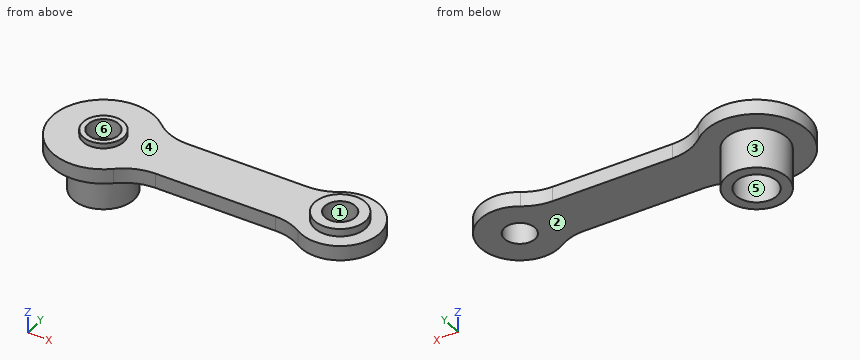
Autodesk Inventor part; units mm, degrees
ref_plane "YZ Plane" through (0, 0, 0) normal (1, 0, 0) x (0, 1, 0)
ref_plane "XZ Plane" through (0, 0, 0) normal (0, 1, 0) x (-1, 0, 0)
ref_plane "XY Plane" through (0, 0, 0) normal (0, 0, 1) x (1, 0, 0)
sketch "Base" plane through (0, 0, 0) normal (0, 0, 1) x (1, 0, 0)
  circle A0 centre (0, 0) radius 10
  line L0 (0, 0) -> (46, 0) construction
  circle A1 centre (46, 0) radius 7.75
  line L1 (8.6603, 5) -> (40.0786, 5)
  line L2 (40.0786, 5) -> (40.0786, -5)
  line L3 (40.0786, -5) -> (8.6603, -5)
  line L4 (8.6603, -5) -> (8.6603, 5)
  circle A2 centre (46, 0) radius 3
  circle A3 centre (0, 0) radius 3
  point P0 (8.6603, 0)
  point P1 (8.6603, -5)
  dimension "d0" = 20
  dimension "d2" = 15.5
  dimension "d1" = 46
  dimension "d3" = 10
  dimension "d4" = 6
  dimension "d5" = 6
extrude "Plate1" add sketch "Base" along normal blind 2.9
sketch "Shoulder" plane through (0, 0, 0) normal (0, 0, -1) x (-1, 0, 0)
  circle A0 centre (0, 0) radius 3
  circle A1 centre (0, 0) radius 3
  circle A2 centre (0, 0) radius 6
  circle A3 centre (0, 0) radius 4
  dimension "d7" = 12
  dimension "d8" = 2
extrude "ShoulderFeature" add sketch "Shoulder" along normal blind 8 contours A2
sketch "Mount" plane through (0, 0, 2.9) normal (0, 0, 1) x (1, 0, 0)
  circle A0 centre (46, 0) radius 3
  circle A1 centre (46, 0) radius 5
  point P0 (0, 0)
  dimension "d11" = 2
extrude "MountFeature" add sketch "Mount" along normal blind 1.5
fillet "BaseFilletsFeature" radius 10 2 edges at (8.6603, 5, 1.45) (8.6603, -5, 1.45)
fillet "EndFilletsFeature" radius 10 2 edges at (40.0786, 5, 1.45) (40.0786, -5, 1.45)
sketch "Sketch6" plane through (0, 0, 2.9) normal (0, 0, 1) x (1, 0, 0)
  circle A0 centre (0, 0) radius 3
  circle A1 centre (0, 0) radius 4
  dimension "d17" = 1
extrude "Extrusion3" add sketch "Sketch6" along normal blind 1
equation "\"d6\" = Thickness"
equation "\"BendRadius\" = Thickness"
equation "\"BendReliefWidth\" = Thickness"
equation "\"BendReliefDepth\" = 0.5 * Thickness"
equation "\"CornerReliefSize\" = 4 * Thickness"
equation "\"MinimumRemnant\" = 2 * Thickness"
equation "\"TransitionRadius\" = BendRadius"
equation "\"JacobiRadiusSize\" = BendRadius"
equation "\"GapSize\" = Thickness"
properties part number "LegChainTensionerArm"
CAD build for the part. Positions are in the model's coordinates, mm. Face numbers are marked on the shaded views. A direction names the side the tool comes from. Coordinates: 2 decimals unless noted, no trailing zeros. Order: outer loops, then holes, each group sorted by start corner. A loop starts at its lowest first (then second) coordinate and runs counter-clockwise, first axis right, second up.
Item 1: Band-saw the part on A-A on x = 46. List the corners of the cut face in (y, z), plus the area to 4 significant figures.
Check sheet entries:
outline: (-7.75, 0) - (-3, 0) - (-3, 4.4) - (-5, 4.4) - (-5, 2.9) - (-7.75, 2.9) - close; (3, 0) - (7.75, 0) - (7.75, 2.9) - (5, 2.9) - (5, 4.4) - (3, 4.4) - close
area: 33.55 mm2
Item 2: Band-saw the part on D-D on x = 0. List the corners of the cut face in (y, z), plus the area to 3 significant figures.
Check sheet entries:
outline: (-10, 0) - (-6, 0) - (-6, -8) - (-4, -8) - (-4, 0) - (-3, 0) - (-3, 3.9) - (-4, 3.9) - (-4, 2.9) - (-10, 2.9) - close; (3, 0) - (4, 0) - (4, -8) - (6, -8) - (6, 0) - (10, 0) - (10, 2.9) - (4, 2.9) - (4, 3.9) - (3, 3.9) - close
area: 74.6 mm2
Item 3: Band-saw the part on B-B on y = 0. List the corners of the cut face in (x, z), plus the area to 3 significant figures.
Check sheet entries:
outline: (-10, 0) - (-6, 0) - (-6, -8) - (-4, -8) - (-4, 0) - (-3, 0) - (-3, 3.9) - (-4, 3.9) - (-4, 2.9) - (-10, 2.9) - close; (3, 0) - (4, 0) - (4, -8) - (6, -8) - (6, 0) - (43, 0) - (43, 4.4) - (41, 4.4) - (41, 2.9) - (4, 2.9) - (4, 3.9) - (3, 3.9) - close; (49, 0) - (53.75, 0) - (53.75, 2.9) - (51, 2.9) - (51, 4.4) - (49, 4.4) - close
area: 190 mm2
Item 4: Drill centre lines: L1, parallel to Y at x = 46, z = 1; L2, parallel to Y at x = 0, z = 0.85; L3, parallel to Z at x = 29, y = -4.5. Where is each one in solid material? Low to high.
Check sheet entries:
L1: y = -7.75 to -3, 3 to 7.75
L2: y = -10 to -3, 3 to 10
L3: z = 0 to 2.9
Item 5: 3-axis set-ups, long thin cutter, end or side, ignore diameter. For the marked faces 4, 5 and 6: which of +Z, -Z, +X, -X, +Y, -Y reach the whole face in a straight line?
Check sheet entries:
face 4: +Z
face 5: -Z
face 6: +Z, -Z
Item 6: Two-plate mould, pull along X, no slides. Class the marked faces 1, 2 and 3: +X half, -X half, draft (parallel to the pull), parting line (faces both ways), or undercut.
Check sheet entries:
face 1: undercut
face 2: draft
face 3: parting line
Item 7: Pin check, flat tips, straight feed: pin 1 Ø9 at (x, y) = (0, 1.5) entering from +Z; pin 2 Ø10 at (x, y) = (19.5, 2.5) entering from -Z; pin 3 Ø5.5 at (x, y) = (46, 0) entering from +Z; pin 4 Ø6 at (x, y) = (24.5, 4) entering from +Z. Stop position of each tip, or through.
Check sheet entries:
pin 1: stops at z = 3.9
pin 2: stops at z = 0
pin 3: passes through
pin 4: stops at z = 2.9
Item 8: Band-saw the part on C-C on z = -5.25. List the corners of the cut face in (x, y), plus the area to 3 significant figures.
Check sheet entries:
outline: circle Ø12 at (0, 0); hole circle Ø8 at (0, 0)
area: 62.8 mm2
